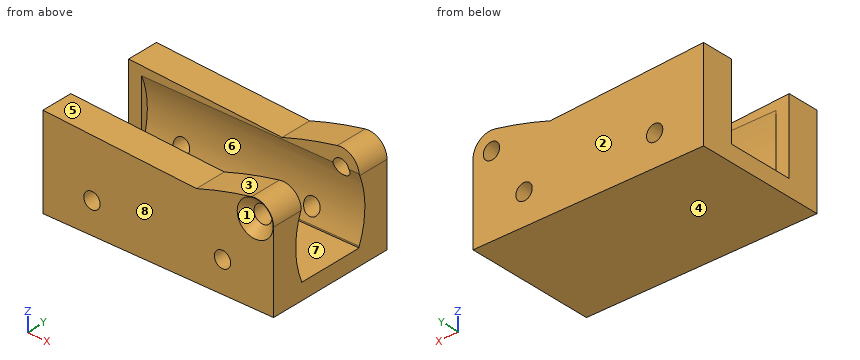
```python
from build123d import *

# Parameters (mm, degrees)
PAD040_DEPTH         = 20
SKETCH138_W          = 20.4
SKETCH138_H          = 70
POCKET051_DEPTH      = 65.001
POCKET051_DEPTH_BACK = 5.651
SKETCH135_R          = 2.5
POCKET049_DEPTH      = 40.001
HOLE028_D            = 5.5
HOLE028_DEPTH        = 20
HOLE028_CSINK_D      = 11
HOLE028_CSINK_ANGLE  = 90
HOLE028_TIPS_R       = 2.75
POCKET050_DEPTH      = 66.651
SKETCH140_R          = 2.5
POCKET054_DEPTH      = 20.001
POCKET054_DEPTH_BACK = 20.001


with BuildPart() as part:
    # Sketch134 → Pad040 (new body, symmetric)
    with BuildSketch(Plane.XZ):
        with BuildLine():
            Line((-18, 1), (-65, 3.5))
            Line((-65, 3.5), (-65, -24.5))
            Line((-65, -24.5), (5.65, -24.5))
            Line((5.65, -24.5), (5.65, 0))
            ThreePointArc((5.65, 0), (3.593093, 4.360296), (-1.079976, 5.545823))
            ThreePointArc((-1.079976, 5.545823), (-9.619729, 3.569716), (-18, 1))
        make_face()
    extrude(amount=PAD040_DEPTH, both=True)

    # Sketch138 → Pocket051 (cut, two sides)
    with BuildSketch(Plane.YZ) as pocket051_sk:
        with Locations((0, 15.5)):
            Rectangle(SKETCH138_W, SKETCH138_H)
    extrude(amount=-POCKET051_DEPTH, mode=Mode.SUBTRACT)
    extrude(pocket051_sk.sketch, amount=POCKET051_DEPTH_BACK, mode=Mode.SUBTRACT)

    # Sketch135 → Pocket049 (cut, through all)
    with BuildSketch(Plane.XZ.offset(20)):
        Circle(SKETCH135_R)
    extrude(amount=-POCKET049_DEPTH, mode=Mode.SUBTRACT)

    # Hole028
    with Locations(Plane.XZ.offset(20)):
        with Locations((0, 0)):
            CounterSinkHole(HOLE028_D / 2, HOLE028_CSINK_D / 2, depth=HOLE028_DEPTH, counter_sink_angle=HOLE028_CSINK_ANGLE)

    # Hole028 tips → Hole028 tip 1 section 0
    with BuildSketch(Plane.XZ, mode=Mode.PRIVATE) as hole028_tip_1_s0:
        Circle(HOLE028_TIPS_R)
    loft([hole028_tip_1_s0.sketch, Vertex(0, 1.652367, 0)], mode=Mode.SUBTRACT)

    # Sketch137 → Pocket050 (cut, through all)
    with BuildSketch(Plane.YZ.offset(-61)):
        with BuildLine():
            ThreePointArc((-10, 1), (-12.197862, -9.25), (-10, -19.5))
            Line((10, -19.5), (-10, -19.5))
            ThreePointArc((10, -19.5), (12.197862, -9.25), (10, 1))
            Line((-10, 1), (10, 1))
        make_face()
    extrude(amount=POCKET050_DEPTH, mode=Mode.SUBTRACT)

    # Sketch140 → Pocket054 (cut, two sides)
    with BuildSketch(Plane.XZ) as pocket054_sk:
        with Locations((-10, -15)):
            Circle(SKETCH140_R)
        with Locations((-50, -15)):
            Circle(SKETCH140_R)
    extrude(amount=-POCKET054_DEPTH, mode=Mode.SUBTRACT)
    extrude(pocket054_sk.sketch, amount=POCKET054_DEPTH_BACK, mode=Mode.SUBTRACT)


solid = part.part
```
Can you work these out from the model? Positions are in its coordinate system, mm. Face numbers are marked on the shaded views. A direction names the side the tool comes from. Give positions to 0.01 mm unless a question says otherwise; leave off trailing zeros. Write each loop counter-clockwise with the first axis right and the second up, starting at its lowest first coordinate (ties: lowest second). Pieces come first, ordered by that corner, then holes. Notation, with made-up numbers: (12.25, 39) - (46.25, 39) arc R21 ccw to (46.25, 53) - close; hole circle Ø6 at (35.5, -35.75). An arc over 180 degrees is marked (long way). Write item = value, one per line. Start each with the question number.
1. Imagine slicing it at B-B (x = 0). Please give me the cut outline in (y, z), and give its area (3 significant figures).
2. For pin 1 (1 mm diameter, centred on x = -9, y = -8.5, fed in from +Z); pin 2 (8 mm diameter, centred on x = -10, z = -15, fed in from -Y); pin 3 (1.6 mm diameter, centred on y = -11, z = -9.5, fed in from +X); pin 4 (1 mm diameter, centred on x = -11, y = -13, fed in from +Z), each with a flat end and sliding along its axis, tell me the tip position at first contact or that it passes through.
3. Imagine slicing it at A-A (y = -16). Please give me the cut outline in (x, z), and give its area (3 significant figures).
4. Imagine slicing it at C-C (z = -15). Please give me the cut outline in (x, y).
5. On a 3-axis mill with a long thin cutter (end or side, diameter ignored), from which of +Z, -Z, +X, -X, +Y, -Y can I reach the whole of each face in a straight line? I mean the marked faces 4, 5, 6, 7 and 8. Say none if no direction works.
6. Please list where these lines run through material, in increasing order: line 1 (X direction, y = -17, z = -15); line 2 (X direction, y = -12.5, z = 0); line 3 (Y direction, x = -58, z = 1).
7. Imagine slicing it at D-D (x = -13.5). Please give me the cut outline in (y, z), and give its area (3 significant figures).
8. Thinking about a two-plate mould opening in Z: for the marked faces 1, 2 and 3, which applies, released by +Z, released by -Z, zero draft, split by the parting line, or undercut?
Worked answers:
q1.outline = (-20, -24.5) - (20, -24.5) - (20, -2.5) - (11.27, -2.5) arc R25 cw to (10.2, -19.04) - (10.2, -19.5) - (-10.2, -19.5) - (-10.2, -19.04) arc R25 cw to (-11.34, -2.75) - (-17.25, -2.75) - (-20, -5.5) - close; (-20, 5.5) - (-17.25, 2.75) - (-10.2, 2.75) - (-10.2, 5.65) - (-20, 5.65) - close; (10.2, 2.5) - (20, 2.5) - (20, 5.65) - (10.2, 5.65) - close
q1.area = 534 mm2
q2.pin_1 = -19.5
q2.pin_2 = -20
q2.pin_3 = -61
q2.pin_4 = 3.33
q3.outline = (-65, -24.5) - (5.65, -24.5) - (5.65, 0) arc R5.65 ccw to (-1.08, 5.55) arc R125 ccw to (-18, 1) - (-65, 3.5) - close; hole circle Ø5 at (-50, -15); hole circle Ø5 at (-10, -15); hole circle Ø5.5 at (0, 0)
q3.area = 1,860 mm2
q4.outline = (-65, -20) - (-52.5, -20) - (-52.5, -11.53) - (-61, -11.53) - (-61, -10.2) - (-65, -10.2) - close; (-65, 10.2) - (-61, 10.2) - (-61, 11.53) - (-52.5, 11.53) - (-52.5, 20) - (-65, 20) - close; (-47.5, -20) - (-12.5, -20) - (-12.5, -11.53) - (-47.5, -11.53) - close; (-47.5, 11.53) - (-12.5, 11.53) - (-12.5, 20) - (-47.5, 20) - close; (-7.5, -20) - (5.65, -20) - (5.65, -11.53) - (-7.5, -11.53) - close; (-7.5, 11.53) - (5.65, 11.53) - (5.65, 20) - (-7.5, 20) - close
q5.face_4 = -Z, +X, -X, +Y, -Y
q5.face_5 = +Z, +Y, -Y
q5.face_6 = +X
q5.face_7 = +Z, +X, -X
q5.face_8 = +Z, -Z, +X, -X, -Y
q6.line_1 = -65 to -52.5, -47.5 to -12.5, -7.5 to 5.65
q6.line_2 = -65 to -2.75, 2.75 to 5.65
q6.line_3 = -20 to -10.2, 10.2 to 20
q7.outline = (-20, -24.5) - (20, -24.5) - (20, 2.46) - (10.2, 2.46) - (10.2, 0.54) arc R25 cw to (10.2, -19.04) - (10.2, -19.5) - (-10.2, -19.5) - (-10.2, -19.04) arc R25 cw to (-10.2, 0.54) - (-10.2, 2.46) - (-20, 2.46) - close
q7.area = 578 mm2
q8.face_1 = undercut
q8.face_2 = zero draft
q8.face_3 = released by +Z
